Design review of the part built by this model. Coordinates are the model's own, in mm. A direction names the side the tool comes from. Round coordinates to 2 decimals unless told otherwise and drop trailing zeros. Loops run counter-clockwise (first coordinate to the right, second up) from the corner with the lowest first, then second, coordinate; pieces in that order, holes last. Notation, with made-up numbers: M 18.5,5 L 28.5,5 A25 ccw 28.5,44 Z; hole C 33,-19.75 d7. An arc over 180 degrees is marked long. One line per item, written item: value. Start each with the question number.
Item 1: For faces 4 (the flat face through (3.8, 9.7, 10.2)), 5 (the flat face through (4, 0.5, 6.6)), 6 (the flat face through (-8, 2.125, -4)), 7 (the flat face through (-8, 5, -3.5)), list the 3-axis set-ups (+Z, -Z, +X, -X, +Y, -Y) from which the entire face can be reached by the end or side of a thin tool; tool diameter is ignored.
Item 2: We need section C-C (z = 9). Write out the cut boundary in (x, y), then the cut area to 3 significant figures.
Item 3: We need section B-B (y = 1.75). Write out the cut boundary in (x, z), then the cut area to 3 significant figures.
Item 4: We need section D-D (y = 5). Write out the cut boundary in (x, z).
Item 5: For line 1 along X through (y, z) = (1, 9.25); line 2 along Z through (x, y) = (-7.75, 2); line 3 along Y through (x, z) = (5.5, -3), list the stretches that pass through material, from the lowest coordinate up.
Item 6: Mouldability with a two-part tool opening along Z and no side actions: class faces 1 (the flat face through (-5, 5, -5.5)), 2 (the flat face through (3.5, 5, 7)), 3 (the flat face through (4, 9.5, 6.6)) as released by +Z, released by -Z, zero draft, split by the parting line, or undercut.
Item 7: We need section A-A (x = -7). Write out the cut boundary in (y, z) (3 decimals).
Item 8: Clearance check with flat-ended pins moving along their axes: pin 1 (1 mm diameter, centred on y = 1.5, z = 10.5, fed in from -X); pin 2 (0.8 mm diameter, centred on y = 5.5, z = -4, fed in from +X); pin 3 (4.5 mm diameter, centred on x = -9.5, y = 6, fed in from +Z). State where each tip first meets the part, or that it passes through.
from build123d import *

# Parameters (mm, degrees)
BOSS_EXTRUDE1_DEPTH = 10
SKETCH2_W           = 7.75
SKETCH2_H           = 5.75
BOSS_EXTRUDE2_DEPTH = 1
CUT_EXTRUDE1_DEPTH  = 28.299267389
CUT_EXTRUDE2_START  = -2
CUT_EXTRUDE2_DEPTH  = 2.8
CUT_EXTRUDE3_START  = -7
CUT_EXTRUDE3_DEPTH  = 2.8


with BuildPart() as part:
    # Sketch1 → Boss-Extrude1 (new body)
    with BuildSketch(Plane(origin=(0, 0, 0), x_dir=(1, 0, 0), z_dir=(0, 1, 0))):
        with BuildLine():
            Line((-15, 4.5), (0, 4.5))
            Line((0, 4.5), (0, 3.5))
            ThreePointArc((0, 3.5), (2.474873734, 2.474873734), (3.5, 0))
            Line((3.5, 0), (3.5, -15))
            Line((3.5, -15), (7.5, -15))
            Line((7.5, -15), (7.5, 2.017195282))
            ThreePointArc((7.5, 2.017195282), (6.594493755, 4.366365807), (4.346513054, 5.5))
            Line((4.346513054, 5.5), (-15, 5.5))
            Line((-15, 5.5), (-15, 4.5))
        make_face()
    extrude(amount=BOSS_EXTRUDE1_DEPTH)

    # Sketch2 → Boss-Extrude2 (add)
    with BuildSketch(Plane.XY.offset(-4.5)):
        with Locations((-7.675, 5)):
            Rectangle(SKETCH2_W, SKETCH2_H)
    extrude(amount=BOSS_EXTRUDE2_DEPTH)

    # Sketch3 → Cut-Extrude1 (cut, through all)
    with BuildSketch(Plane.XY.offset(15)):
        with BuildLine():
            Line((7.5, 7.8), (7.5, 2.2))
            ThreePointArc((7.5, 2.2), (4.7, 5), (7.5, 7.8))
        make_face()
    extrude(amount=-CUT_EXTRUDE1_DEPTH, mode=Mode.SUBTRACT)

    # Sketch4 → Cut-Extrude2 (cut)
    with BuildSketch(Plane.XY.offset(15).offset(CUT_EXTRUDE2_START)):
        Polygon((4.5, 10), (3.5, 9), (3.5, 10), align=None)
        Polygon((3.5, 1), (3.5, 0), (4.5, 0), align=None)
    extrude(amount=-CUT_EXTRUDE2_DEPTH, mode=Mode.SUBTRACT)

    # Sketch4<2> → Cut-Extrude3 (cut)
    with BuildSketch(Plane.XY.offset(15).offset(CUT_EXTRUDE3_START)):
        Polygon((4.5, 10), (3.5, 9), (3.5, 10), align=None)
        Polygon((3.5, 1), (3.5, 0), (4.5, 0), align=None)
    extrude(amount=-CUT_EXTRUDE3_DEPTH, mode=Mode.SUBTRACT)


solid = part.part
A:
1. face 4: -X, +Y
1. face 5: -X, -Y
1. face 6: +Z, -X, -Y
1. face 7: +Z, -X, +Y, -Y
2. outline: M 3.5,0 L 7.5,0 L 7.5,2.2 A2.8 cw 7.5,7.8 L 7.5,10 L 3.5,10 Z
2. area: 27.7 mm2
3. outline: M -15,-5.5 L 4.35,-5.5 A3.5 ccw 7.5,-2.02 L 7.5,15 L 3.5,15 L 3.5,0 A3.5 cw 0,-3.5 L 0,-4.5 L -15,-4.5 Z
3. area: 104 mm2
4. outline: M -15,-5.5 L 4.35,-5.5 A3.5 ccw 4.7,-5.45 L 4.7,15 L 3.5,15 L 3.5,0 A3.5 cw 0,-3.5 L 0,-4.5 L -3.8,-4.5 L -3.8,-3.5 L -11.55,-3.5 L -11.55,-4.5 L -15,-4.5 Z
5. line 1: 3.5 to 7.5
5. line 2: -5.5 to -4.5
5. line 3: 0 to 3.04, 6.96 to 10
6. face 1: released by -Z
6. face 2: zero draft
6. face 3: undercut
7. outline: M 0,-5.5 L 10,-5.5 L 10,-4.5 L 7.875,-4.5 L 7.875,-3.5 L 2.125,-3.5 L 2.125,-4.5 L 0,-4.5 Z
8. pin 1: x = 3.5
8. pin 2: x = 4.85
8. pin 3: z = -3.5
